Autodesk Inventor part; units mm, degrees
ref_plane "YZ Plane" through (0, 0, 0) normal (1, 0, 0) x (0, 1, 0)
ref_plane "XZ Plane" through (0, 0, 0) normal (0, 1, 0) x (-1, 0, 0)
ref_plane "XY Plane" through (0, 0, 0) normal (0, 0, 1) x (1, 0, 0)
sketch "Sketch1" plane through (0, 0, 0) normal (0, 1, 0) x (-1, 0, 0)
  line L0 (7.493, 14.986) -> (-7.493, 14.986)
  line L1 (-7.493, 14.986) -> (-7.493, -14.986)
  line L2 (-7.493, -14.986) -> (7.493, -14.986)
  line L3 (7.493, -14.986) -> (7.493, 14.986)
  line L4 (7.493, 14.986) -> (-7.493, -14.986) construction
  line L5 (-7.493, 14.986) -> (7.493, -14.986) construction
  point P0 (0, 0)
  dimension "d0" = 29.972
  dimension "d1" = 14.986
extrude "Extrusion1" add sketch "Sketch1" along normal blind 7.366
sketch "Sketch2" plane through (0, 0, 0) normal (1, 0, 0) x (0, 1, 0)
  line L0 (7.366, 14.986) -> (7.366, -14.986)
  line L1 (7.366, 10.16) -> (22.352, 10.16)
  arc A0 (22.352, -10.16) -> (22.352, 10.16) centre (22.352, 0) ccw
  line L2 (22.352, -10.16) -> (7.366, -10.16)
  line L3 (7.366, 10.16) -> (7.366, -10.16)
  circle A1 centre (22.352, 0) radius 5.08
  point P0 (0, 0)
  dimension "d4" = 14.986
  dimension "d5" = 10.16
  dimension "d6" = 10.16
  dimension "d7" = 10.16
extrude "Extrusion2" add sketch "Sketch2" along normal mid plane 7.366
fillet "Fillet1" radius 1.016 7 edges at (7.493, 3.683, 14.986) (7.493, 7.366, 0) (7.493, 3.683, -14.986) (0, 7.366, -14.986) (0, 7.366, 14.986) (-7.493, 3.683, 14.986) (-7.493, 7.366, 0)
fillet "Fillet2" radius 1.016 6 edges at (3.683, 32.512, 0) (3.683, 14.859, -10.16) (3.683, 14.859, 10.16) (-3.683, 32.512, 0) (-3.683, 14.859, -10.16) (-3.683, 14.859, 10.16)
fillet "Fillet3" radius 1.016 8 edges at (3.3854, 7.366, 9.8624) (0, 7.366, 10.16) (-3.3854, 7.366, 9.8624) (-3.683, 7.366, 0) (-3.3854, 7.366, -9.8624) (0, 7.366, -10.16) (3.3854, 7.366, -9.8624) (3.683, 7.366, 0)
fillet "Fillet4" radius 1.016 2 edges at (-7.1954, 7.0684, -14.6884) (-7.493, 3.175, -14.986)
properties part number "Pivot"
CAD build for the part. Positions are in the model's coordinates, mm. A direction names the side the tool comes from. Round coordinates to 2 decimals unless told otherwise and drop trailing zeros. Loops run counter-clockwise (first coordinate to the right, second up) from the corner with the lowest first, then second, coordinate; pieces in that order, holes last. Notation, with made-up numbers: (66.5, -32) - (84.5, -32) arc R36 cw to (84.5, 2) - close; hole circle Ø1 at (37.25, 89). An arc over 180 degrees is marked (long way). Return JSON: item names as keys, results as strings. Group by question number.
Q1. Two-plate mould, pull along Y, no slides. Class faces 6 (the face through (0, 0, 0)), 7 (the face through (3.393, 15.465, -9.854)), 8 (the face through (-0.05, 18.32, 3.09)), 9 (the face through (-0.091, 7.076, -14.68)): +Y half, -Y half, draft (parallel to the pull), parting line (faces both ways), or undercut.
Q2. Tool access for faces 1 (the face through (3.683, 17, 0)), 2 (the face through (0, 15, -10.16)), 3 (the face through (-3.38, 15.46, -9.87)), 4 (the face through (0, 15, 10.16)), 5 (the face through (6, 7.366, 0)): list every direction of +Z, -Z, +X, -X, +Y, -Y with a clear straight run to the whole face (end or side of a thin tool).
Q3. Band-saw the part on B-B on y = 20.5. Give the cut face in (x, z).
Q4. Band-saw the part on C-C on z = 0. Give the cut face in (x, y), plus the area to 3 significant figures.
Q5. Drill centre lines: line 1 along Y through (x, z) = (-4.75, 3.25); line 2 along X through (y, z) = (28, 2.5); line 3 along Z through (x, y) = (1, 10.5). Where is each one in solid material? Low to high. Write a range as [from, to].
Q6. Band-saw the part on D-D on y = 11.5. Give the cut face in (x, z), plus the area to 3 significant figures.
Q7. Band-saw the part on A-A on x = 1.5. Give the cut face in (y, z).
Q8. Flat gauge pins, fed straight in: pin 1 Ø6 at (x, y) = (-5.5, 16) entering from -Z; pin 2 Ø14.5 at (y, z) = (25, -1.5) entering from -X; pin 3 Ø4.5 at (x, y) = (0, 18) entering from +Z. Where does each tip first touch, or does it go through?
Solutions:
{
 "1": {"face 6": "-Y half", "face 7": "draft", "face 8": "undercut", "face 9": "+Y half"},
 "2": {"face 1": "+Z, -Z, +X, +Y", "face 2": "-Z, +X, -X, +Y", "face 3": "-Z, -X, +Y", "face 4": "+Z, +X, -X, +Y", "face 5": "+Y"},
 "3": {"outline": "(-3.68, -9.14) arc R1.02 ccw to (-2.67, -10.16) - (2.67, -10.16) arc R1.02 ccw to (3.68, -9.14) - (3.68, -4.73) - (-3.68, -4.73) - close; (-3.68, 4.73) - (3.68, 4.73) - (3.68, 9.14) arc R1.02 ccw to (2.67, 10.16) - (-2.67, 10.16) arc R1.02 ccw to (-3.68, 9.14) - close"},
 "4": {"outline": "(-7.49, 0) - (7.49, 0) - (7.49, 6.35) arc R1.02 ccw to (6.48, 7.37) - (4.7, 7.37) arc R1.02 cw to (3.68, 8.38) - (3.68, 17.27) - (-3.68, 17.27) - (-3.68, 8.38) arc R1.02 cw to (-4.7, 7.37) - (-6.48, 7.37) arc R1.02 ccw to (-7.49, 6.35) - close; (-3.68, 27.43) - (3.68, 27.43) - (3.68, 31.5) arc R1.02 ccw to (2.67, 32.51) - (-2.67, 32.51) arc R1.02 ccw to (-3.68, 31.5) - close", "area": "220 mm^2"},
 "5": {"line 1": "y = [0, 7.37]", "line 2": "x = [-3.68, 3.68]", "line 3": "z = [-10.16, 10.16]"},
 "6": {"outline": "(-3.68, -9.14) arc R1.02 ccw to (-2.67, -10.16) - (2.67, -10.16) arc R1.02 ccw to (3.68, -9.14) - (3.68, 9.14) arc R1.02 ccw to (2.67, 10.16) - (-2.67, 10.16) arc R1.02 ccw to (-3.68, 9.14) - close", "area": "149 mm^2"},
 "7": {"outline": "(0, -14.99) - (6.35, -14.99) arc R1.02 ccw to (7.37, -13.97) - (7.37, -11.18) arc R1.02 cw to (8.38, -10.16) - (22.35, -10.16) arc R10.16 ccw to (22.35, 10.16) - (8.38, 10.16) arc R1.02 cw to (7.37, 11.18) - (7.37, 13.97) arc R1.02 ccw to (6.35, 14.99) - (0, 14.99) - close; hole circle Ø10.16 at (22.35, 0)"},
 "8": {"pin 1": "stops at z = -10.16", "pin 2": "stops at x = -3.68", "pin 3": "stops at z = 10.16"}
}
